The listing builds one solid part. Answer for the finished solid, in the listing's coordinates (mm). Face numbers are marked on the shaded views. Coordinates: 2 decimals unless noted, no trailing zeros. Order: outer loops, then holes, each group sorted by start corner. A loop starts at its lowest first (then second) coordinate and runs counter-clockwise, first axis right, second up.
```python
from build123d import *

# Parameters (mm, degrees)
SKETCH1_R           = 1.65
BOSS_EXTRUDE1_DEPTH = 1.3
DEBURS_SIZE         = 0.2


with BuildPart() as part:
    # Sketch1 → Boss-Extrude1 (new, symmetric)
    with BuildSketch(Plane.XY):
        Polygon((2.7, -1.558845727), (2.7, 1.558845727), (0, 3.117691454), (-2.7, 1.558845727), (-2.7, -1.558845727), (0, -3.117691454), align=None)
        Circle(SKETCH1_R, mode=Mode.SUBTRACT)
    extrude(amount=BOSS_EXTRUDE1_DEPTH, both=True)

    # Deburs
    deburs_edges = [part.edges().sort_by_distance(p)[0] for p in [
        (1.35, 2.33826859, 1.3),
        (-1.35, 2.33826859, 1.3),
        (-1.65, 0, -1.3),
        (-1.65, 0, 1.3),
        (-2.7, 0, 1.3),
        (-1.35, -2.33826859, 1.3),
        (1.35, -2.33826859, 1.3),
        (-1.35, -2.33826859, -1.3),
        (-2.7, 0, -1.3),
        (-1.35, 2.33826859, -1.3),
        (1.35, 2.33826859, -1.3),
        (2.7, 0, -1.3),
        (1.35, -2.33826859, -1.3),
        (2.7, 0, 1.3),
    ]]
    chamfer(deburs_edges, length=DEBURS_SIZE)


solid = part.part
```
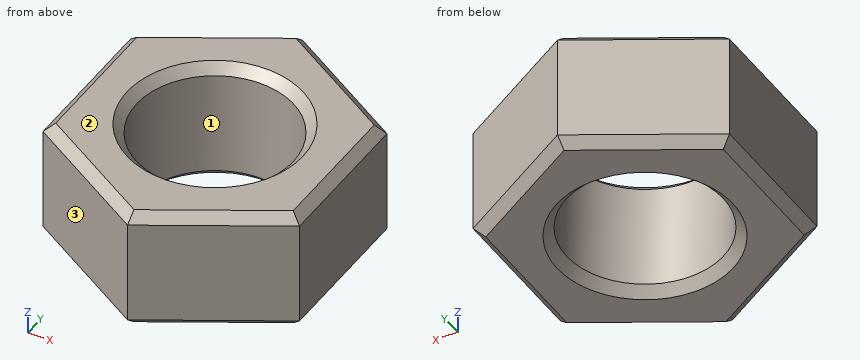
1) A cutting plane is placed at C-C, the plane y = 2. Write down the section's boundary in (x, z).
2) A cutting plane is placed at B-B, the plane z = -0.5. Write down the section's boundary in (x, y).
3) A cutting plane is placed at D-D, the plane y = -2.5. Write down the section's boundary in (x, z), plus the area to 3 significant figures.
4) The mould has two halves that part along X. Classify the marked faces 1, 2 and 3: released by +X, released by -X, zero draft, split by the parting line, or undercut.
5) A cutting plane is placed at A-A, the plane y = 0. Write down the section's boundary in (x, z).
6) Straight lines are drawn through the part: probe 1 along Y at (x, z) = (-0.2, 0); probe 2 along X at (y, z) = (0.5, 0.5); probe 3 along X at (y, z) = (-0.75, -0.95). For each, find the intervals that lie inside material, in ascending order.
7) Each of these flat-tipped pins is pushed along its axis until it touches: P1, Ø3, axis at x = 0, y = 0, coming from the +Z side; P2, Ø3, axis at x = 0, y = 1, coming from the -Z side; P3, Ø1, axis at x = 1, z = -0.5, coming from the +Y side. Where does it stop, or does it pass through?
Working result:
1. outline: (-1.94, -1.1) - (-1.54, -1.3) - (1.54, -1.3) - (1.94, -1.1) - (1.94, 1.1) - (1.54, 1.3) - (-1.54, 1.3) - (-1.94, 1.1) - close
2. outline: (-2.7, -1.56) - (0, -3.12) - (2.7, -1.56) - (2.7, 1.56) - (0, 3.12) - (-2.7, 1.56) - close; hole circle Ø3.3 at (0, 0)
3. outline: (-1.07, -1.1) - (-0.67, -1.3) - (0.67, -1.3) - (1.07, -1.1) - (1.07, 1.1) - (0.67, 1.3) - (-0.67, 1.3) - (-1.07, 1.1) - close
3. area: 5.40 mm2
4. face 1: undercut
4. face 2: zero draft
4. face 3: released by -X
5. outline: (-2.7, -1.1) - (-2.5, -1.3) - (-1.85, -1.3) - (-1.65, -1.1) - (-1.65, 1.1) - (-1.85, 1.3) - (-2.5, 1.3) - (-2.7, 1.1) - close; (1.65, -1.1) - (1.85, -1.3) - (2.5, -1.3) - (2.7, -1.1) - (2.7, 1.1) - (2.5, 1.3) - (1.85, 1.3) - (1.65, 1.1) - close
6. probe 1: y = -3 to -1.64, 1.64 to 3
6. probe 2: x = -2.7 to -1.57, 1.57 to 2.7
6. probe 3: x = -2.7 to -1.47, 1.47 to 2.7
7. P1: passes through
7. P2: stops at z = -1.3
7. P3: stops at y = 2.83
